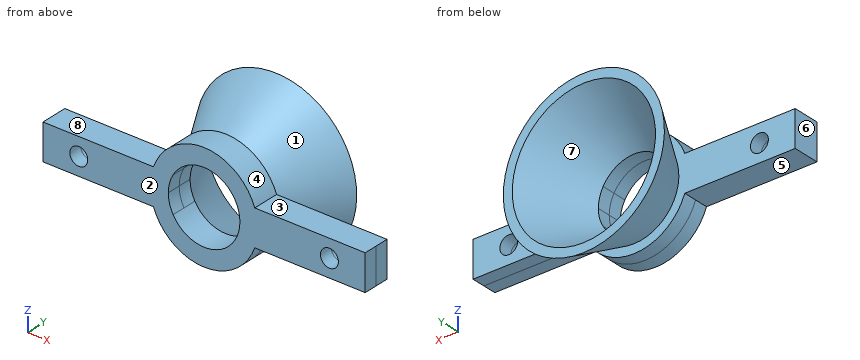
```python
from build123d import *

# Parameters (mm, degrees)
SKETCH1_R           = 0.79375
BOSS_EXTRUDE1_DEPTH = 1.190625


with BuildPart() as part:
    # Sketch1 → Boss-Extrude1 (new, symmetric)
    # profile 1 of 14: a face of its own
    with BuildSketch(Plane(origin=(0, 0, 0), x_dir=(1, 0, 0), z_dir=(0, 1, 0))):
        with BuildLine():
            ThreePointArc((-4.682314967, -0.870248702), (-4.742411374, -0.436967517), (-4.7625, 0))
            ThreePointArc((-4.7625, 0), (-4.69391314, 0.805348174), (-4.490128061, 1.5875))
            Line((-4.490128061, 1.5875), (-14.2875, 1.5875))
            Line((-14.2875, 1.5875), (-14.2875, -1.5875))
            Line((-14.2875, -1.5875), (-5.924630657, -1.5875))
            Line((-5.924630657, -1.5875), (-4.682314967, -0.870248702))
        make_face()
        with Locations(Location((-11.1125, 0, 0), (0, 0, 90))):
            Circle(SKETCH1_R, mode=Mode.SUBTRACT)
    # profile 2 of 14: a face of its own
    with BuildSketch(Plane(origin=(0, 0, 0), x_dir=(1, 0, 0), z_dir=(0, 1, 0))):
        with BuildLine():
            ThreePointArc((-2.749630657, 1.5875), (0, 3.175), (2.749630657, 1.5875))
            Line((2.749630657, 1.5875), (4.490128061, 1.5875))
            ThreePointArc((4.490128061, 1.5875), (0, 4.7625), (-4.490128061, 1.5875))
            Line((-4.490128061, 1.5875), (-2.749630657, 1.5875))
        make_face()
    # profile 3 of 14: a face of its own
    with BuildSketch(Plane(origin=(0, 0, 0), x_dir=(1, 0, 0), z_dir=(0, 1, 0))):
        with BuildLine():
            ThreePointArc((4.490128061, 1.5875), (4.69391314, 0.805348174), (4.7625, 0))
            ThreePointArc((4.7625, 0), (4.742411374, -0.436967517), (4.682314967, -0.870248702))
            Line((4.682314967, -0.870248702), (5.924630657, -1.5875))
            Line((5.924630657, -1.5875), (14.2875, -1.5875))
            Line((14.2875, -1.5875), (14.2875, 1.5875))
            Line((14.2875, 1.5875), (4.490128061, 1.5875))
        make_face()
        with Locations(Location((11.1125, 0, 0), (0, 0, 90))):
            Circle(SKETCH1_R, mode=Mode.SUBTRACT)
    # profile 4 of 14: a face of its own
    with BuildSketch(Plane(origin=(0, 0, 0), x_dir=(1, 0, 0), z_dir=(0, 1, 0))):
        with BuildLine():
            ThreePointArc((2.749630657, 1.5875), (3.066814498, 0.821750468), (3.175, 0))
            Line((3.175, 0), (4.7625, 0))
            ThreePointArc((4.7625, 0), (4.69391314, 0.805348174), (4.490128061, 1.5875))
            Line((4.490128061, 1.5875), (2.749630657, 1.5875))
        make_face()
    # profile 5 of 14: a face of its own
    with BuildSketch(Plane(origin=(0, 0, 0), x_dir=(1, 0, 0), z_dir=(0, 1, 0))):
        with BuildLine():
            Line((-4.7625, 0), (-3.175, 0))
            ThreePointArc((-3.175, 0), (-3.066814498, 0.821750468), (-2.749630657, 1.5875))
            Line((-2.749630657, 1.5875), (-4.490128061, 1.5875))
            ThreePointArc((-4.490128061, 1.5875), (-4.69391314, 0.805348174), (-4.7625, 0))
        make_face()
    # profile 6 of 14: a face of its own
    with BuildSketch(Plane(origin=(0, 0, 0), x_dir=(1, 0, 0), z_dir=(0, 1, 0))):
        with BuildLine():
            Line((4.7625, 0), (3.175, 0))
            Line((3.175, 0), (4.682314967, -0.870248702))
            ThreePointArc((4.682314967, -0.870248702), (4.742411374, -0.436967517), (4.7625, 0))
        make_face()
    # profile 7 of 14: a face of its own
    with BuildSketch(Plane(origin=(0, 0, 0), x_dir=(1, 0, 0), z_dir=(0, 1, 0))):
        with BuildLine():
            Line((4.682314967, -0.870248702), (3.175, 0))
            ThreePointArc((3.175, 0), (3.066814498, -0.821750468), (2.749630657, -1.5875))
            Line((2.749630657, -1.5875), (4.490128061, -1.5875))
            ThreePointArc((4.490128061, -1.5875), (4.600221748, -1.232625702), (4.682314967, -0.870248702))
        make_face()
    # profile 8 of 14: a face of its own
    with BuildSketch(Plane(origin=(0, 0, 0), x_dir=(1, 0, 0), z_dir=(0, 1, 0))):
        with BuildLine():
            Line((4.490128061, -1.5875), (2.749630657, -1.5875))
            ThreePointArc((2.749630657, -1.5875), (0, -3.175), (-2.749630657, -1.5875))
            Line((-2.749630657, -1.5875), (-4.490128061, -1.5875))
            ThreePointArc((-4.490128061, -1.5875), (0, -4.7625), (4.490128061, -1.5875))
        make_face()
    # profile 9 of 14: a face of its own
    with BuildSketch(Plane(origin=(0, 0, 0), x_dir=(1, 0, 0), z_dir=(0, 1, 0))):
        with BuildLine():
            ThreePointArc((-2.749630657, -1.5875), (-3.066814498, -0.821750468), (-3.175, 0))
            Line((-3.175, 0), (-4.682314967, -0.870248702))
            ThreePointArc((-4.682314967, -0.870248702), (-4.600221748, -1.232625702), (-4.490128061, -1.5875))
            Line((-4.490128061, -1.5875), (-2.749630657, -1.5875))
        make_face()
    # profile 10 of 14: a face of its own
    with BuildSketch(Plane(origin=(0, 0, 0), x_dir=(1, 0, 0), z_dir=(0, 1, 0))):
        with BuildLine():
            ThreePointArc((2.749630657, 1.5875), (3.066814498, 0.821750468), (3.175, 0))
            Line((3.175, 0), (4.7625, 0))
            ThreePointArc((4.7625, 0), (4.69391314, 0.805348174), (4.490128061, 1.5875))
            Line((4.490128061, 1.5875), (2.749630657, 1.5875))
        make_face()
    # profile 11 of 14: a face of its own
    with BuildSketch(Plane(origin=(0, 0, 0), x_dir=(1, 0, 0), z_dir=(0, 1, 0))):
        with BuildLine():
            Line((-4.7625, 0), (-3.175, 0))
            ThreePointArc((-3.175, 0), (-3.066814498, 0.821750468), (-2.749630657, 1.5875))
            Line((-2.749630657, 1.5875), (-4.490128061, 1.5875))
            ThreePointArc((-4.490128061, 1.5875), (-4.69391314, 0.805348174), (-4.7625, 0))
        make_face()
    # profile 12 of 14: a face of its own
    with BuildSketch(Plane(origin=(0, 0, 0), x_dir=(1, 0, 0), z_dir=(0, 1, 0))):
        with BuildLine():
            Line((-4.682314967, -0.870248702), (-3.175, 0))
            Line((-3.175, 0), (-4.7625, 0))
            ThreePointArc((-4.7625, 0), (-4.742411374, -0.436967517), (-4.682314967, -0.870248702))
        make_face()
    # profile 13 of 14: a face of its own
    with BuildSketch(Plane(origin=(0, 0, 0), x_dir=(1, 0, 0), z_dir=(0, 1, 0))):
        with BuildLine():
            Line((5.924630657, -1.5875), (4.682314967, -0.870248702))
            ThreePointArc((4.682314967, -0.870248702), (4.600221748, -1.232625702), (4.490128061, -1.5875))
            Line((4.490128061, -1.5875), (5.924630657, -1.5875))
        make_face()
    # profile 14 of 14: a face of its own
    with BuildSketch(Plane(origin=(0, 0, 0), x_dir=(1, 0, 0), z_dir=(0, 1, 0))):
        with BuildLine():
            ThreePointArc((-4.490128061, -1.5875), (-4.600221748, -1.232625702), (-4.682314967, -0.870248702))
            Line((-4.682314967, -0.870248702), (-5.924630657, -1.5875))
            Line((-5.924630657, -1.5875), (-4.490128061, -1.5875))
        make_face()
    extrude(amount=BOSS_EXTRUDE1_DEPTH, both=True)

    # Sketch2 → Revolve2 (revolve)
    with BuildSketch(Plane.XY, mode=Mode.PRIVATE) as revolve2_sk:
        Polygon((-3.175, 1.190625), (-6.35, 6.689886314), (-7.14375, 6.689886314), (-3.96875, 1.190625), align=None)
    revolve(revolve2_sk.sketch.rotate(Axis((0, -1000, 0), (0, 1, 0)), 270), axis=Axis((0, -1000, 0), (0, 1, 0)))


solid = part.part
```
Part model, mm, in its own coordinate system. Face numbers are marked on the shaded views. A direction names the side the tool comes from. Give positions to 0.01 mm unless a question says otherwise; leave off trailing zeros. Write each loop counter-clockwise with the first axis right and the second up, starting at its lowest first coordinate (ties: lowest second). Pieces come first, ordered by that corner, then holes. Notation, with made-up numbers: (-4.75, 28.25) -> (39.25, 28.25) arc R29 cw to (39.25, 67.25) -> close; hole circle Ø4 at (33.25, 32). An arc over 180 degrees is marked (long way). Put each result on its own line as item: value. Start each with the question number.
Item 1: Wall check: L1, parallel to Y at x = 9, z = -1; L2, parallel to X at y = 6, z = 1.75; L3, parallel to Z at x = -7.25, y = 0. Give the ranges that are in metal, low to high. Write a range as [from, to].
Item 2: Cut at C-C (x = -7.5). List the corners of the cut face in (y, z).
Item 3: Which spindle directions (+Z, -Z, +X, -X, +Y, -Y) get a long thin tool onto all of the face, cutting with end or side? Do the marked faces 1, 2, 3 and 4. Say none if no direction does.
Item 4: Pin check, flat tips, straight feed: pin 1 Ø1.3 at (x, y) = (8.5, 0.5) entering from -Z; pin 2 Ø2.5 at (x, y) = (-11.5, -0.5) entering from +Z; pin 3 Ø3 at (y, z) = (6, 2) entering from +X; pin 4 Ø1.3 at (x, z) = (11.11, 0) entering from +Y. Stop position of each tip, or through.
Item 5: Cut at B-B (z = -0.5). State how many separate pieces and enclosed holes the cut face has, then the cut area to 3 significant figures.
Item 6: Pull direction Z, two halves, no side cores. Call the marked faces 5, 6, 7 and 8: pulls with the +Z half, pulls with the -Z half, needs draft (parallel to the pull), parting line crosses it, or undercut.
Answer list:
1. L1: y = [-1.19, 1.19]
1. L2: x = [-6.51, -5.69], [5.69, 6.51]
1. L3: z = [-1.59, 1.59]
2. outline: (-1.19, -1.59) -> (1.19, -1.59) -> (1.19, 1.59) -> (-1.19, 1.59) -> close
3. face 1: none
3. face 2: +Z, -Z, +X, -X, -Y
3. face 3: +Z, +X, -Y
3. face 4: +Z, -Y
4. pin 1: stops at z = -1.59
4. pin 2: stops at z = 1.59
4. pin 3: stops at x = 7.11
4. pin 4: passes through
5. separate pieces: 4
5. enclosed holes: 0
5. area: 56.0 mm2
6. face 5: pulls with the -Z half
6. face 6: needs draft
6. face 7: undercut
6. face 8: pulls with the +Z half
